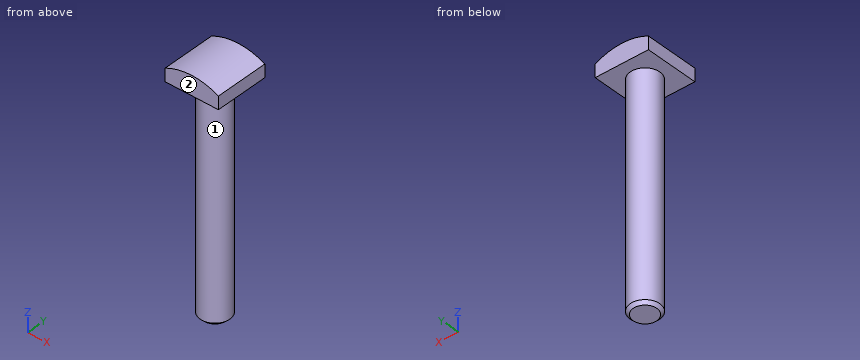
Solid Edge part; units mm, degrees
sketch "Sketch1" plane through (0, 0, 0) normal (0, 0, 1) x (1, 0, 0)
  line L0 (-9, -9) -> (9, -9)
  line L1 (9, -9) -> (9, 9)
  line L2 (9, 9) -> (-9, 9)
  line L3 (-9, 9) -> (-9, -9)
extrude "Protrusion1" add sketch "Sketch1" along normal mid plane 6.5
sketch "Sketch2" plane through (0, 0, -3.25) normal (0, 0, -1) x (1, 0, 0)
  circle A0 centre (0, 0) radius 5
extrude "ExtrudedProtrusion_2" add sketch "Sketch2" along normal blind 75 and the other way blind 35.9412
sketch "Sketch3" plane through (0, -9, 0) normal (0, -1, 0) x (1, 0, 0)
  line L0 (23.9875, 3.25) -> (23.9875, 36.6911)
  line L1 (23.9875, 36.6911) -> (-10.6415, 36.6911)
  line L2 (-10.6415, 36.6911) -> (-10.6415, 3.25)
  line L3 (-10.6415, 3.25) -> (9, 3.25)
  line L4 (9, 3.25) -> (23.9875, 3.25)
extrude "Cutout1" cut sketch "Sketch3" against normal through all and the other way through all
cosmetic_thread "Thread_1" thread depth 26
chamfer "Chamfer_1" distance 1 angle 45 1 edges at (-5, 0, -78.25)
sketch "Sketch4" plane through (0, -9, 0) normal (0, -1, 0) x (1, 0, 0)
  line L0 (-14.1953, 12.3388) -> (14.0888, 12.3388)
  line L1 (14.0888, 12.3388) -> (14.0888, -2.5547)
  arc A0 (-14.1953, -2.6612) -> (14.0888, -2.5547) centre (0, -16.75) cw
  line L2 (-14.1953, -2.6612) -> (-14.1953, 12.3388)
extrude "ExtrudedCutout_3" cut sketch "Sketch4" against normal blind 36.133 and the other way blind 1.0534
Source: CAD feature listing. Evaluate the final solid. Frame: model axes, mm. Face numbers are marked on the shaded views. A direction names the side the tool comes from. Give positions to 0.01 mm unless a question says otherwise; leave off trailing zeros. Write each loop counter-clockwise with the first axis right and the second up, starting at its lowest first coordinate (ties: lowest second). Pieces come first, ordered by that corner, then holes. Notation, with made-up numbers: M 42,-11.5 L 100,-11.5 A34 ccw 100,22.5 Z; hole C 22.5,-8 d8. An arc over 180 degrees is marked long. Return JSON: item names as keys, results as strings. Group by question number.
1) Cut plane C-C, the plane z = -32. Output: boundary loops of the cut face in (x, y), then the cut area to 3 significant figures.
2) Cut plane B-B, the plane y = 0. Output: boundary loops of the cut face in (x, z), then the cut area to 3 significant figures.
3) Ray query, L1, parallel to Z at x = -0.25, y = 2.5; L2, parallel to Z at x = 0.75, y = 6; L3, parallel to Y at x = 0.25, z = -13.5. Return the intervals inside material, ascending.
4) Cut plane D-D, the plane x = 6. Output: boundary loops of the cut face in (y, z).
5) Cut plane A-A, the plane x = 0. Output: boundary loops of the cut face in (y, z), then the cut area to 3 significant figures.
6) First-contact query: pin 1 Ø8 at (y, z) = (-3, -70) entering from -X; pin 2 Ø5 at (x, z) = (7, -8) entering from -Y; pin 3 Ø3 at (y, z) = (6, -12.5) entering from +X. Flat tips, straight axial feed; report the tip coordinate or a pass-through.
7) Set-up query: the marked faces 1 and 2. Return all of +Z, -Z, +X, -X, +Y, -Y with unobstructed straight access to the full face (end or side cutting, diameter ignored); none if empty.
Data:
{
 "1": {"outline": "C 0,0 d10", "area": "78.5 mm²"},
 "2": {"outline": "M -9,-3.25 L -5,-3.25 L -5,-77.25 L -4,-78.25 L 4,-78.25 L 5,-77.25 L 5,-3.25 L 9,-3.25 L 9,1.11 A20 ccw -9,1.11 Z", "area": "853 mm²"},
 "3": {"L1": "z = -78.25 to 3.25", "L2": "z = -3.25 to 3.24", "L3": "y = -4.99 to 4.99"},
 "4": {"outline": "M -9,-3.25 L 9,-3.25 L 9,2.33 L -9,2.33 Z"},
 "5": {"outline": "M -9,-3.25 L -5,-3.25 L -5,-77.25 L -4,-78.25 L 4,-78.25 L 5,-77.25 L 5,-3.25 L 9,-3.25 L 9,3.25 L -9,3.25 Z", "area": "866 mm²"},
 "6": {"pin 1": "stops at x = -5", "pin 2": "stops at y = -2.18", "pin 3": "stops at x = 2.18"},
 "7": {"face 1": "-Z", "face 2": "+Z, -Z, +X, -X, -Y"}
}
